Could you check a few things on this model? Use its own coordinates, in mm. Give positions to 0.01 mm unless a question says otherwise; leave off trailing zeros. Order: outer loops, then holes, each group sorted by start corner. A loop starts at its lowest first (then second) coordinate and runs counter-clockwise, first axis right, second up. Notation, with made-up numbers: (70.25, 63) -> (82.25, 63) arc R16 cw to (82.25, 76) -> close; hole circle Ø4 at (70.5, 77.5). An arc over 180 degrees is marked (long way). Write each question's results on one line, items separated by ' | '.
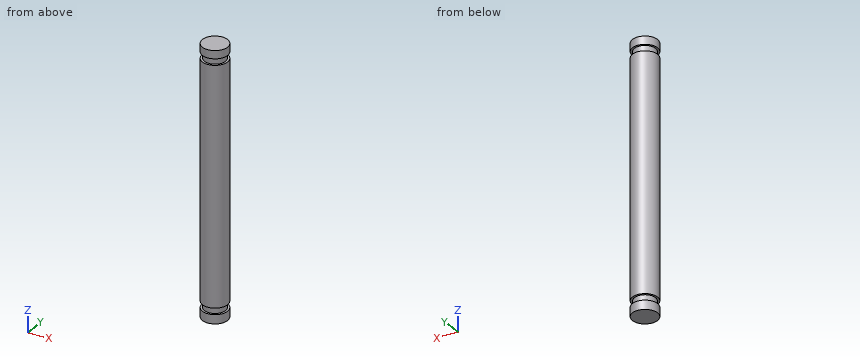
```python
from build123d import *

# Parameters (mm, degrees)
SKETCH1_R           = 3.175
BOSS_EXTRUDE1_DEPTH = 59.6138
SKETCH2_R           = 2.667
BOSS_EXTRUDE2_DEPTH = 1.6002
SKETCH3_R           = 3.175
BOSS_EXTRUDE3_DEPTH = 2.286
SKETCH4_R           = 2.667
BOSS_EXTRUDE4_DEPTH = 1.6002
SKETCH5_R           = 3.175
BOSS_EXTRUDE5_DEPTH = 2.032


with BuildPart() as part:
    # Sketch1 → Boss-Extrude1 (new body)
    with BuildSketch(Plane.XY):
        Circle(SKETCH1_R)
    extrude(amount=BOSS_EXTRUDE1_DEPTH)

    # Sketch2 → Boss-Extrude2 (add)
    with BuildSketch(Plane(origin=(0, 0, 0), x_dir=(-1, 0, 0), z_dir=(0, 0, -1))):
        Circle(SKETCH2_R)
    extrude(amount=BOSS_EXTRUDE2_DEPTH)

    # Sketch3 → Boss-Extrude3 (add)
    with BuildSketch(Plane(origin=(0, 0, -1.6002), x_dir=(-1, 0, 0), z_dir=(0, 0, -1))):
        Circle(SKETCH3_R)
    extrude(amount=BOSS_EXTRUDE3_DEPTH)

    # Sketch4 → Boss-Extrude4 (add)
    with BuildSketch(Plane.XY.offset(59.6138)):
        Circle(SKETCH4_R)
    extrude(amount=BOSS_EXTRUDE4_DEPTH)

    # Sketch5 → Boss-Extrude5 (add)
    with BuildSketch(Plane.XY.offset(61.214)):
        Circle(SKETCH5_R)
    extrude(amount=BOSS_EXTRUDE5_DEPTH)


solid = part.part
```
Q1. I need wall thicknesses on line 1 along Z through (x, y) = (-3, -0.75); line 2 along X through (y, z) = (-0.25, 32); line 3 along X through (y, z) = (2, 46). Which ranges of each line are inside material? Lowest first, please.
Here are the results:
line 1: z = -3.89 to -1.6, 0 to 59.61, 61.21 to 63.25 | line 2: x = -3.17 to 3.17 | line 3: x = -2.47 to 2.47
Q2. Suppose I cut it at C-C on y = 1.5. Please give me the cut outline in (x, z), and give its area (3 significant figures).
Here are the results:
outline: (-2.8, -3.89) -> (2.8, -3.89) -> (2.8, -1.6) -> (2.21, -1.6) -> (2.21, 0) -> (2.8, 0) -> (2.8, 59.61) -> (2.21, 59.61) -> (2.21, 61.21) -> (2.8, 61.21) -> (2.8, 63.25) -> (-2.8, 63.25) -> (-2.8, 61.21) -> (-2.21, 61.21) -> (-2.21, 59.61) -> (-2.8, 59.61) -> (-2.8, 0) -> (-2.21, 0) -> (-2.21, -1.6) -> (-2.8, -1.6) -> close | area: 372 mm²
Q3. I'm going to push flat-ended pins straight in: pin 1 Ø1 at (y, z) = (1, 45) entering from +X; pin 2 Ø1 at (x, z) = (-2, 48) entering from +Y; pin 3 Ø2 at (y, z) = (-2, 7) entering from +X. Where does each tip first touch, or does it pass through?
Here are the results:
pin 1: stops at x = 3.14 | pin 2: stops at y = 2.8 | pin 3: stops at x = 3.01
Q4. Suppose I cut it at B-B on z = 17. Please give me the cut outline in (x, y) (3 decimals).
Here are the results:
outline: circle Ø6.35 at (0, 0)
Q5. Suppose I cut it at A-A on x = -0.5. Please give me the cut outline in (y, z), and give its area (3 significant figures).
Here are the results:
outline: (-3.14, -3.89) -> (3.14, -3.89) -> (3.14, -1.6) -> (2.62, -1.6) -> (2.62, 0) -> (3.14, 0) -> (3.14, 59.61) -> (2.62, 59.61) -> (2.62, 61.21) -> (3.14, 61.21) -> (3.14, 63.25) -> (-3.14, 63.25) -> (-3.14, 61.21) -> (-2.62, 61.21) -> (-2.62, 59.61) -> (-3.14, 59.61) -> (-3.14, 0) -> (-2.62, 0) -> (-2.62, -1.6) -> (-3.14, -1.6) -> close | area: 418 mm²
